```python
from build123d import *

# Parameters (mm, degrees)
SKETCH_1_R      = 1.5
SKETCH_1_R_2    = 3
EXTRUDE_1_DEPTH = 2.5
SKETCH_2_R      = 4.85
SKETCH_2_R_2    = 3
EXTRUDE_2_DEPTH = 5


with BuildPart() as part:
    # 草图1 → 凸台-拉伸1 (new body)
    with BuildSketch(Plane.XY):
        with BuildLine():
            Line((-0.343, -4.887980258), (-20.245, -3.49141447))
            ThreePointArc((-20.245, -3.49141447), (-23.5, 0), (-20.245, 3.49141447))
            Line((-20.245, 3.49141447), (-0.343, 4.887980258))
            ThreePointArc((-0.343, 4.887980258), (0, 4.9), (0.343, 4.887980258))
            Line((0.343, 4.887980258), (20.245, 3.49141447))
            ThreePointArc((20.245, 3.49141447), (23.5, 0), (20.245, -3.49141447))
            Line((20.245, -3.49141447), (0.343, -4.887980258))
            ThreePointArc((0.343, -4.887980258), (0, -4.9), (-0.343, -4.887980258))
        make_face()
        with Locations((20, 0)):
            Circle(SKETCH_1_R, mode=Mode.SUBTRACT)
        with Locations((16, 0)):
            Circle(SKETCH_1_R, mode=Mode.SUBTRACT)
        with Locations((12, 0)):
            Circle(SKETCH_1_R, mode=Mode.SUBTRACT)
        Circle(SKETCH_1_R_2, mode=Mode.SUBTRACT)
        with Locations(Location((-12, 0, 0), (0, 0, 180))):
            Circle(SKETCH_1_R, mode=Mode.SUBTRACT)
        with Locations(Location((-16, 0, 0), (0, 0, 180))):
            Circle(SKETCH_1_R, mode=Mode.SUBTRACT)
        with Locations(Location((-20, 0, 0), (0, 0, 180))):
            Circle(SKETCH_1_R, mode=Mode.SUBTRACT)
    extrude(amount=EXTRUDE_1_DEPTH)

    # 草图2 → 凸台-拉伸2 (add)
    with BuildSketch(Plane.XY.offset(2.5)):
        Circle(SKETCH_2_R)
        Circle(SKETCH_2_R_2, mode=Mode.SUBTRACT)
    extrude(amount=EXTRUDE_2_DEPTH)


solid = part.part
```
The model under review builds one solid part; all positions refer to its coordinate system, in mm. A direction names the side the tool comes from. Round coordinates to 2 decimals unless told otherwise and drop trailing zeros. Loops run counter-clockwise (first coordinate to the right, second up) from the corner with the lowest first, then second, coordinate; pieces in that order, holes last. Notation, with made-up numbers: (30, -40) - (70, -40) arc R23 cw to (70, -26) - close; hole circle Ø8 at (53.25, -30.75). An arc over 180 degrees is marked (long way). Use a Markdown table: item, result. Add a question column.
Q1. Add section B-B (z = 0.5). State the section outline as (x, y) points (3 decimals).
Q2. Add section D-D (z = 4.25). State the section outline as (x, y) points.
Q3. The part is to be moulded in two halves that separate along Y. For faces 3 (the face through (10.43, -4.18, 1.23)), 4 (the face through (10.15, 4.2, 1.23)), 5 (the face through (-10.5, -0.07, 1.23)), 6 (the face through (0.3, -3.2, 0)), say which applies: pulls with the +Y half, pulls with the -Y half, needs draft (parallel to the pull), parting line crosses it, or undercut.
Q4. Machinability: for faces 1 (the face through (4.626, 1.457, 4.965)), 2 (the face through (-23.5, -0.1, 1.2)), which of the approach directions +Z, -Z, +X, -X, +Y, -Y give a long, thin tool a straight path to every point of the face, cutting with its end or side? Answer none if there is none.
Q5. Add section C-C (y = 0). State how many separate pieces and enclosed holes the cut face has, plus the area to 3 significant figures.
Q6. Add section A-A (x = -15). State the section outline as (y, z) points.
Q7. For probe 1 along Z at (x, y) = (17, 2.25); probe 2 along Y at (x, z) = (17, 2); probe 3 along X at (y, z) = (-2.25, 3.5), list the stretches that pass through material, from the lowest coordinate up.
Q8. Insertion check: pin 1 Ø3 at (y, z) = (1, 5.5) entering from +X; pin 2 Ø3 at (y, z) = (-4, 6.5) entering from +X; pin 3 Ø4 at (x, z) = (-10, 1) entering from +Y; pin 4 Ø5 at (x, y) = (-20, 0) entering from -Z. Each pin has a flat end and moves straight along its axis. Give the tip position at first contact, or say it passes through.
Worked answers:
| question | item | result |
|---|---|---|
| 1 | outline | (-20.245, -3.491) - (-0.343, -4.888) arc R4.9 ccw to (0.343, -4.888) - (20.245, -3.491) arc R3.5 ccw to (20.245, 3.491) - (0.343, 4.888) arc R4.9 ccw to (-0.343, 4.888) - (-20.245, 3.491) arc R3.5 ccw to start; hole circle Ø3 at (-20, 0); hole circle Ø3 at (-16, 0); hole circle Ø3 at (-12, 0); hole circle Ø6 at (0, 0); hole circle Ø3 at (12, 0); hole circle Ø3 at (16, 0); hole circle Ø3 at (20, 0) |
| 2 | outline | circle Ø9.7 at (0, 0); hole circle Ø6 at (0, 0) |
| 3 | face 3 | pulls with the -Y half |
| 3 | face 4 | pulls with the +Y half |
| 3 | face 5 | undercut |
| 3 | face 6 | needs draft |
| 4 | face 1 | +Z |
| 4 | face 2 | +Z, -Z, -X |
| 5 | separate pieces | 8 |
| 5 | enclosed holes | 0 |
| 5 | area | 76.0 mm² |
| 6 | outline | (-3.86, 0) - (-1.12, 0) - (-1.12, 2.5) - (-3.86, 2.5) - close; (1.12, 0) - (3.86, 0) - (3.86, 2.5) - (1.12, 2.5) - close |
| 7 | probe 1 | 0 to 2.5 |
| 7 | probe 2 | -3.72 to -1.12, 1.12 to 3.72 |
| 7 | probe 3 | -4.3 to -1.98, 1.98 to 4.3 |
| 8 | pin 1 | x = 4.85 |
| 8 | pin 2 | x = 4.16 |
| 8 | pin 3 | y = 4.35 |
| 8 | pin 4 | z = 0 |
